```python
from build123d import *

# Parameters (mm, degrees)
SKETCH1_W                = 65
SKETCH1_H                = 100
BOSS_EXTRUDE1_DEPTH      = 3.5
SKETCH2_W                = 40
SKETCH2_H                = 61
CUT_EXTRUDE1_DEPTH       = 1.4
SKETCH3_R                = 2
CUT_EXTRUDE3_DEPTH       = 3.5
SKETCH4_R                = 2
CUT_EXTRUDE5_DEPTH       = 3.5
SKETCH6_R                = 2
CUT_EXTRUDE6_DEPTH       = 3.5
SKETCH7_R                = 2
CUT_EXTRUDE7_DEPTH       = 3.5
SKETCH9_W                = 19
SKETCH9_H                = 6
CUT_EXTRUDE9_DEPTH       = 2.3
SKETCH10_W               = 22.5
SKETCH10_H               = 4.5
CUT_EXTRUDE10_DEPTH      = 3.5
CUT_EXTRUDE11_DEPTH      = 2.3
CUT_EXTRUDE15_DEPTH      = 2.5
SKETCH18_W               = 2.7
SKETCH18_H               = 50.5
CUT_EXTRUDE18_DEPTH      = 2.5
SKETCH8_W                = 5
SKETCH8_H                = 11.5
CUT_EXTRUDE25_DEPTH      = 3.5
SKETCH20_R               = 7.5
CUT_EXTRUDE27_DEPTH      = 2.4
CUT_EXTRUDE27_DEPTH_BACK = 3.1
SKETCH21_W               = 5.3
SKETCH21_H               = 2.85
CUT_EXTRUDE28_DEPTH      = 3.5
CUT_EXTRUDE30_DEPTH      = 3
FILLET2_R                = 0.5
SKETCH27_R               = 6.6
CUT_EXTRUDE32_DEPTH      = 1.5
SKETCH28_W               = 5.5
SKETCH28_H               = 5.5
CUT_EXTRUDE33_DEPTH      = 3
FILLET4_R                = 1


with BuildPart() as part:
    # Sketch1 → Boss-Extrude1 (new body)
    with BuildSketch(Plane(origin=(0, 0, 0), x_dir=(1, 0, 0), z_dir=(0, 1, 0))):
        Rectangle(SKETCH1_W, SKETCH1_H)
    extrude(amount=BOSS_EXTRUDE1_DEPTH)

    # Sketch2 → Cut-Extrude1 (cut)
    with BuildSketch(Plane(origin=(0, 0, 0), x_dir=(1, 0, 0), z_dir=(0, 1, 0))):
        with Locations((-8, 5)):
            Rectangle(SKETCH2_W, SKETCH2_H)
    extrude(amount=CUT_EXTRUDE1_DEPTH, mode=Mode.SUBTRACT)

    # Sketch3 → Cut-Extrude3 (cut)
    with BuildSketch(Plane(origin=(0, 0, 0), x_dir=(1, 0, 0), z_dir=(0, 1, 0))):
        with Locations((-21, 28.5)):
            Circle(SKETCH3_R)
    extrude(amount=CUT_EXTRUDE3_DEPTH, mode=Mode.SUBTRACT)

    # Sketch4 → Cut-Extrude5 (cut)
    with BuildSketch(Plane(origin=(0, 0, 0), x_dir=(1, 0, 0), z_dir=(0, 1, 0))):
        with Locations((5, 28.5)):
            Circle(SKETCH4_R)
    extrude(amount=CUT_EXTRUDE5_DEPTH, mode=Mode.SUBTRACT)

    # Sketch6 → Cut-Extrude6 (cut)
    with BuildSketch(Plane(origin=(0, 0, 0), x_dir=(1, 0, 0), z_dir=(0, 1, 0))):
        with Locations((-25.5, -10)):
            Circle(SKETCH6_R)
    extrude(amount=CUT_EXTRUDE6_DEPTH, mode=Mode.SUBTRACT)

    # Sketch7 → Cut-Extrude7 (cut)
    with BuildSketch(Plane(origin=(0, 0, 0), x_dir=(1, 0, 0), z_dir=(0, 1, 0))):
        with Locations((9.5, -10)):
            Circle(SKETCH7_R)
    extrude(amount=CUT_EXTRUDE7_DEPTH, mode=Mode.SUBTRACT)

    # Sketch9 → Cut-Extrude9 (cut)
    with BuildSketch(Plane(origin=(0, 0, 0), x_dir=(1, 0, 0), z_dir=(0, 1, 0))):
        with Locations((-8, -0.5)):
            Rectangle(SKETCH9_W, SKETCH9_H)
    extrude(amount=CUT_EXTRUDE9_DEPTH, mode=Mode.SUBTRACT)

    # Sketch10 → Cut-Extrude10 (cut)
    with BuildSketch(Plane(origin=(0, 0, 0), x_dir=(1, 0, 0), z_dir=(0, 1, 0))):
        with Locations((-8, -23.25)):
            Rectangle(SKETCH10_W, SKETCH10_H)
    extrude(amount=CUT_EXTRUDE10_DEPTH, mode=Mode.SUBTRACT)

    # Sketch11 → Cut-Extrude11 (cut)
    with BuildSketch(Plane(origin=(0, 0, 0), x_dir=(1, 0, 0), z_dir=(0, 1, 0))):
        Polygon((-28, -25.5), (3.25, -25.5), (12, -25.5), (12, -21), (12, -8), (-28, -8), align=None)
    extrude(amount=CUT_EXTRUDE11_DEPTH, mode=Mode.SUBTRACT)

    # Sketch12 → Cut-Extrude15 (cut)
    with BuildSketch(Plane(origin=(0, 0, 0), x_dir=(1, 0, 0), z_dir=(0, 1, 0))):
        Polygon((28, -20.8), (28, 25), (30.7, 25), (30.7, -25.5), (12, -25.5), (12, -20.8), align=None)
    extrude(amount=CUT_EXTRUDE15_DEPTH, mode=Mode.SUBTRACT)

    # Sketch18 → Cut-Extrude18 (cut)
    with BuildSketch(Plane(origin=(0, 0, 0), x_dir=(1, 0, 0), z_dir=(0, 1, 0))):
        with Locations((-30.15, -0.25)):
            Rectangle(SKETCH18_W, SKETCH18_H)
    extrude(amount=CUT_EXTRUDE18_DEPTH, mode=Mode.SUBTRACT)

    # Sketch8 → Cut-Extrude25 (cut)
    with BuildSketch(Plane(origin=(0, 0, 0), x_dir=(1, 0, 0), z_dir=(0, 1, 0))):
        with Locations((-25.5, -17.95)):
            Rectangle(SKETCH8_W, SKETCH8_H)
    extrude(amount=CUT_EXTRUDE25_DEPTH, mode=Mode.SUBTRACT)

    # Sketch20 → Cut-Extrude27 (cut, two sides)
    with BuildSketch(Plane.XZ.offset(-1.4)) as cut_extrude27_sk:
        with Locations((-7.887877966, -16.952018436)):
            Circle(SKETCH20_R)
    extrude(amount=CUT_EXTRUDE27_DEPTH, mode=Mode.SUBTRACT)
    extrude(cut_extrude27_sk.sketch, amount=-CUT_EXTRUDE27_DEPTH_BACK, mode=Mode.SUBTRACT)

    # Sketch21 → Cut-Extrude28 (cut)
    with BuildSketch(Plane.XZ):
        with Locations((-20.15, -48.575)):
            Rectangle(SKETCH21_W, SKETCH21_H)
        with Locations((20.15, -48.575)):
            Rectangle(SKETCH21_W, SKETCH21_H)
    extrude(amount=-CUT_EXTRUDE28_DEPTH, mode=Mode.SUBTRACT)

    # Sketch25 → Cut-Extrude30 (cut)
    with BuildSketch(Plane.XY.offset(50)):
        Polygon((22.8, 3.5), (13.764153607, 3.5), (12.132076804, 0), (24.432076804, 0), align=None)
        Polygon((-22.8, 3.5), (-24.432076804, 0), (-12.132076804, 0), (-13.764153607, 3.5), align=None)
    extrude(amount=-CUT_EXTRUDE30_DEPTH, mode=Mode.SUBTRACT)

    # Fillet2
    fillet2_edges = [part.edges().sort_by_distance(p)[0] for p in [
        (-15.387877966, 1.4, -16.952018436),
        (-15.387877966, 3.5, -16.952018436),
    ]]
    fillet(fillet2_edges, radius=FILLET2_R)

    # Sketch27 → Cut-Extrude32 (cut)
    with BuildSketch(Plane(origin=(0, 3.5, 0), x_dir=(1, 0, 0), z_dir=(0, 1, 0))):
        with Locations((0, -36.08346839)):
            Circle(SKETCH27_R)
    extrude(amount=-CUT_EXTRUDE32_DEPTH, mode=Mode.SUBTRACT)

    # Sketch28 → Cut-Extrude33 (cut, through all)
    with BuildSketch(Plane(origin=(0, 2, 0), x_dir=(1, 0, 0), z_dir=(0, 1, 0))):
        with Locations((0, -36.08346839)):
            Rectangle(SKETCH28_W, SKETCH28_H)
    extrude(amount=-CUT_EXTRUDE33_DEPTH, mode=Mode.SUBTRACT)

    # Fillet4
    fillet4_edges = [part.edges().sort_by_distance(p)[0] for p in [
        (2.75, 0, 36.08346839),
        (0, 0, 38.83346839),
        (-2.75, 0, 36.08346839),
        (0, 0, 33.33346839),
    ]]
    fillet(fillet4_edges, radius=FILLET4_R)


solid = part.part
```
Could you check a few things on this model? Use its own coordinates, in mm. A direction names the side the tool comes from. Give positions to 0.01 mm unless a question says otherwise; leave off trailing zeros. Order: outer loops, then holes, each group sorted by start corner. A loop starts at its lowest first (then second) coordinate and runs counter-clockwise, first axis right, second up.
Q1. For faces 4 (the flat face through (23.627, 1.726, 48.521)), 5 (the flat face through (12, 1, -7)), 6 (the flat face through (0, 2, 39)), which set-ups out of +Z, -Z, +X, -X, +Y, -Y let a thin tool reach every point of the face, with its end or its side?
Q2. If I drill on line 1 along X through (y, z) = (1.25, 8.5); line 2 along X through (y, z) = (2.75, -28.5); line 3 along Z through (x, y) = (-15.5, 2.1), over which ranges is the centre line in solid material (lowest first)?
Q3. I'm going to push a flat-ended pin straight in: P1, Ø14, axis at x = -12, z = 13, coming from the -Y side. Where does the tip first touch, or does it pass through?
Q4. Suppose I cut it at B-B, the plane x = 5. Write out the boundary of the cut face in (y, z), and give its area (3 significant figures).
Q5. Suppose I cut it at A-A, the plane x = -21. Write out the boundary of the cut face in (y, z), and give its area (3 significant figures).
Q6. We'd pull the mould along Z, two halves only. Please class faces 1 (the flat face through (20, 2, -47.15)), 2 (the flat face through (32.5, 2, 1)), 3 (the flat face through (-8, 2.3, 0)): +Z half, -Z half, draft (parallel to the pull), parting line (faces both ways), or undercut.
Solution:
1. face 4: +Z, -Y
1. face 5: -Y
1. face 6: +Y
2. line 1: x = -32.5 to -31.5, -28.8 to -28, 12 to 28, 30.7 to 32.5
2. line 2: x = -32.5 to -23, -19 to 3, 7 to 32.5
2. line 3: z = -50 to -2.5, 3.5 to 8, 25.5 to 47
3. P1: stops at y = 1.4
4. outline: (0, -50) - (3.5, -50) - (3.5, -30.5) - (1.4, -30.5) - (1.4, -35.5) - (0, -35.5) - close; (0, 25.5) - (2.3, 25.5) - (2.3, 8) - (1.4, 8) - (1.4, -26.5) - (3.5, -26.5) - (3.5, 31.78) - (2, 31.78) - (2, 40.39) - (3.5, 40.39) - (3.5, 50) - (0, 50) - close
4. area: 228 mm2
5. outline: (0, -47.15) - (3.5, -47.15) - (3.5, -30.5) - (1.4, -30.5) - (1.4, -35.5) - (0, -35.5) - close; (0, 25.5) - (2.3, 25.5) - (2.3, 8) - (1.4, 8) - (1.4, -26.5) - (3.5, -26.5) - (3.5, 47) - (0, 47) - close
5. area: 220 mm2
6. face 1: -Z half
6. face 2: draft
6. face 3: undercut
